Part model, mm, in its own coordinate system. A direction names the side the tool comes from. Give positions to 0.01 mm unless a question says otherwise; leave off trailing zeros. Write each loop counter-clockwise with the first axis right and the second up, starting at its lowest first coordinate (ties: lowest second). Pieces come first, ordered by that corner, then holes. Notation, with made-up numbers: (68, 58) - (112, 58) arc R26 cw to (112, 79) - close; hole circle Ø9 at (58.5, 6.5). An arc over 180 degrees is marked (long way). Answer as a JSON object with one key per item and string values. Group by question number.
```python
from build123d import *

# Parameters (mm, degrees)
F0_W     = 11.614211
F0_H     = 105.660983
F0_W_2   = 17.562951
F0_H_2   = 35.975726
F1_DEPTH = 40


with BuildPart() as f1:
    # F0 (on Front) → F1 (new body)
    with BuildSketch(Plane.XZ):
        Polygon((-64.444698, 53.397033), (-64.444698, 45.465384), (-52.830487, 45.465384), (-10.339479, 45.465384), (7.223472, 45.465384), (7.223472, 53.397033), align=None)
        with Locations((-58.637592, -7.365107)):
            Rectangle(F0_W, F0_H)
        with Locations((-1.558003, 27.477521)):
            Rectangle(F0_W_2, F0_H_2)
    extrude(amount=F1_DEPTH)


solid = f1.part
```
1) Probe line 1 (X direction, y = -3, z = 21); line 2 (X direction, y = -13.5, z = -14); line 3 (Z direction, x = -39, y = -34). List the from-to ranges inside material, lowest first.
2) Band-saw the part on A-A (z = 27.5). List the corners of the cut face in (x, y), plus the area to 3 significant figures.
3) Mould opens along X. For faces 4 (the flat face through (-10.339, -20, 27)), 5 (the flat face through (-64.445, -20, 49)), 6 (the flat face through (-28, -20, 53.397)) say: pulls with the +X half, pulls with the -X half, needs draft (parallel to the pull), parting line crosses it, or undercut.
4) Band-saw the part on C-C (x = -51). List the corners of the cut face in (y, z), plus the area to 3 significant figures.
5) Band-saw the part on B-B (y = -9). List the corners of the cut face in (x, z), plus the area to 3 significant figures.
6) Which spindle directions (+Z, -Z, +X, -X, +Y, -Y) get a long thin tool onto all of the face, cutting with end or side? Do faces 1 (the flat face through (-52.83, -20, -8)), 2 (the flat face through (-2, -20, 9.49)), 3 (the flat face through (-59, -20, -60.196)). Say none if no direction does.
7) Band-saw the part on D-D (z = -37). List the corners of the cut face in (x, y), plus the area to 3 significant figures.
8) Drop flat-ended pins along their axis: P1, Ø10, axis at x = -45.5, y = -6.5, coming from the -Z side; P2, Ø8, axis at x = -3.5, y = -14.5, coming from the -Z side. Give the stop position or say it passes through.
Verdict:
{
 "1": {"line 1": "-64.44 to -52.83, -10.34 to 7.22", "line 2": "-64.44 to -52.83", "line 3": "45.47 to 53.4"},
 "2": {"outline": "(-64.44, -40) - (-52.83, -40) - (-52.83, 0) - (-64.44, 0) - close; (-10.34, -40) - (7.22, -40) - (7.22, 0) - (-10.34, 0) - close", "area": "1,170 mm2"},
 "3": {"face 4": "undercut", "face 5": "pulls with the -X half", "face 6": "needs draft"},
 "4": {"outline": "(-40, 45.47) - (0, 45.47) - (0, 53.4) - (-40, 53.4) - close", "area": "317 mm2"},
 "5": {"outline": "(-64.44, -60.2) - (-52.83, -60.2) - (-52.83, 45.47) - (-10.34, 45.47) - (-10.34, 9.49) - (7.22, 9.49) - (7.22, 53.4) - (-64.44, 53.4) - close", "area": "2,430 mm2"},
 "6": {"face 1": "-Z, +Y, -Y", "face 2": "-Z, +X, +Y, -Y", "face 3": "-Z, +X, -X, +Y, -Y"},
 "7": {"outline": "(-64.44, -40) - (-52.83, -40) - (-52.83, 0) - (-64.44, 0) - close", "area": "465 mm2"},
 "8": {"P1": "z = 45.47", "P2": "z = 9.49"}
}
